Work out the finished part from the listing and answer in its coordinate system (mm). Round coordinates to 2 decimals unless told otherwise and drop trailing zeros. Write each loop counter-clockwise with the first axis right and the second up, starting at its lowest first coordinate (ties: lowest second). Pieces come first, ordered by that corner, then holes. Notation, with made-up numbers: (-9, 12.5) -> (-3, 12.5) arc R22 ccw to (-3, 36.5) -> close; hole circle Ø3 at (82.25, -36.75). An arc over 180 degrees is marked (long way). One line per item, written item: value.
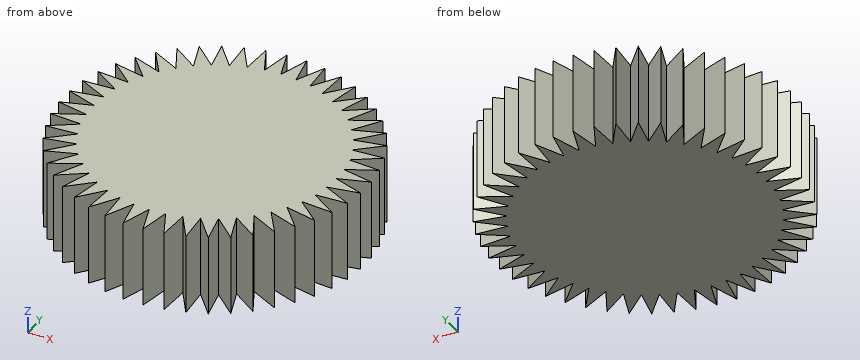
```python
from build123d import *

# Parameters (mm, degrees)
PAD_DEPTH          = 8
POLARPATTERN_COUNT = 48


with BuildPart() as part:
    # Sketch → Pad (new body)
    with BuildSketch(Plane.XY):
        with BuildLine():
            ThreePointArc((0, 12.0248747975), (-0.7864644404, -11.9991286175), (1.5695611192, 11.9220003266))
            Line((1.5695611192, 11.9220003266), (0.982673828, 14.9927053872))
            Line((0, 12.0248747975), (0.982673828, 14.9927053872))
        make_face()
    extrude(amount=PAD_DEPTH)

    # PolarPattern: part ×48 about axis
    polarpattern_axis = Axis((0, 0, 0), (0, 0, 1))


with BuildPart() as part_1:
    add(part.part)
    for i in range(1, POLARPATTERN_COUNT):
        add(part.part.rotate(polarpattern_axis, i * 360 / POLARPATTERN_COUNT))


solid = part_1.part
```
(1) Consider probe 1 along X at (y, z) = (10.75, 7.5); probe 2 along Y at (x, z) = (11.5, 3.75); probe 3 along X at (y, z) = (-11, 1.75). Determine where each line is inside the solid, lowest interval first.
Reported:
probe 1: x = -9.63 to -9.1, -7.74 to -6.39, -6.08 to 6.08, 6.39 to 7.74, 9.1 to 9.63
probe 2: y = -8 to -7.23, -6.24 to -4.94, -4.63 to 4.63, 4.94 to 6.24, 7.23 to 8
probe 3: x = -9.76 to -9.47, -7.83 to -6.67, -6.13 to 6.13, 6.67 to 7.83, 9.47 to 9.76
(2) Flat-ended cylindrical pins translate along their axes: pin 1 Ø3 at (y, z) = (11, 1.5) entering from -X; pin 2 Ø4 at (x, z) = (-7.5, 6.5) entering from -Y; pin 3 Ø1.5 at (y, z) = (1.5, 1) entering from -X. Find the tip coordinate at first contact, or state that the pin passes through.
Reported:
pin 1: stops at x = -11.3
pin 2: stops at y = -13.48
pin 3: stops at x = -14.99
(3) Find section A-A on y = -13. Give the number of separate pieces and of enclosed holes in the cut face, plus the area to 3 significant figures.
Reported:
separate pieces: 8
enclosed holes: 0
area: 48.2 mm2
(4) Find section D-D on y = 0.5. Give the vertices of the cut face in (x, z).
Reported:
outline: (-13.53, 0) -> (13.53, 0) -> (13.53, 8) -> (-13.53, 8) -> close
(5) Find section B-B on y = -8. Give the vertices of the cut face in (x, z).
Reported:
outline: (-12.18, 0) -> (-11.49, 0) -> (-11.49, 8) -> (-12.18, 8) -> close; (-10, 0) -> (10, 0) -> (10, 8) -> (-10, 8) -> close; (11.49, 0) -> (12.18, 0) -> (12.18, 8) -> (11.49, 8) -> close
(6) Find section C-C on x = 2.5. Give the vertices of the cut face in (y, z), plus the area to 3 significant figures.
Reported:
outline: (-13.84, 0) -> (13.84, 0) -> (13.84, 8) -> (-13.84, 8) -> close
area: 222 mm2
